Here's the drawing with two shaded views (mm, measured from the low corner). I have some questions. Coordinates: 2 decimals unless noted, no trailing zeros. Order: outer loops, then holes, each group sorted by start corner. A loop starts at its lowest first (then second) coordinate and runs counter-clockwise, first axis right, second up. Notation, with made-up numbers: (59, 65) -> (97, 65) arc R11 ccw to (97, 81) -> close; hole circle Ø4 at (13, 15). An arc over 180 degrees is marked (long way). Write item = value, one per line.
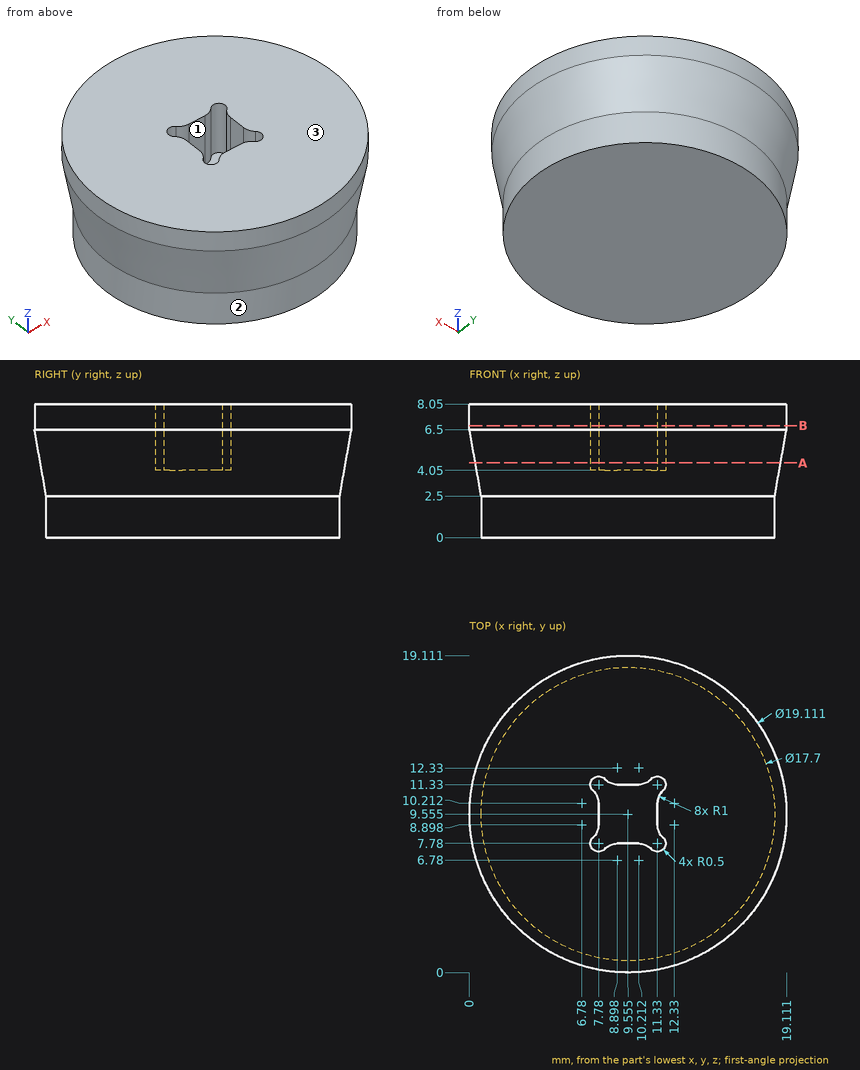
Item 1: I want a section at B-B, the plane z = 6.75. Please give me the cut outline in (x, y) (1 decimal).
A:
outline = circle Ø19.1 at (9.6, 9.6); hole (7.4, 8.2) arc R0.5 ccw (long way) to (8.2, 7.4) arc R1 cw to (8.9, 7.8) -> (10.2, 7.8) arc R1 cw to (11, 7.4) arc R0.5 ccw (long way) to (11.7, 8.2) arc R1 cw to (11.3, 8.9) -> (11.3, 10.2) arc R1 cw to (11.7, 11) arc R0.5 ccw (long way) to (11, 11.7) arc R1 cw to (10.2, 11.3) -> (8.9, 11.3) arc R1 cw to (8.2, 11.7) arc R0.5 ccw (long way) to (7.4, 11) arc R1 cw to (7.8, 10.2) -> (7.8, 8.9) arc R1 cw to start
Item 2: I'm going to push flat-ended pins straight in: P1, Ø3, axis at x = 17, z = 2.5, coming from the +Y side; P2, Ø1.1, axis at x = 9.5, z = 5, coming from the -Y side; P3, Ø1.5, axis at x = 4.5, z = 1, coming from the -Y side. Where does each tip first touch, or does it pass through?
A:
P1 = 16.16
P2 = 0.17
P3 = 1.82
Item 3: If I drill on probe 1 along X at (y, z) = (9.5, 4.75); probe 2 along X at (y, z) = (9.25, 4.5); probe 3 along Y at (x, z) = (11, 5) (1 decimal), over which ranges is the centre line in solid material (lowest first)?
A:
probe_1 = 0.31 to 7.78, 11.33 to 18.8
probe_2 = 0.36 to 7.78, 11.33 to 18.75
probe_3 = 0.4 to 7.4, 11.7 to 18.7
Item 4: I want a section at A-A, the plane z = 4.5. Please give me the cut outline in (x, y) (1 decimal).
A:
outline = circle Ø18.4 at (9.6, 9.6); hole (7.4, 8.2) arc R0.5 ccw (long way) to (8.2, 7.4) arc R1 cw to (8.9, 7.8) -> (10.2, 7.8) arc R1 cw to (11, 7.4) arc R0.5 ccw (long way) to (11.7, 8.2) arc R1 cw to (11.3, 8.9) -> (11.3, 10.2) arc R1 cw to (11.7, 11) arc R0.5 ccw (long way) to (11, 11.7) arc R1 cw to (10.2, 11.3) -> (8.9, 11.3) arc R1 cw to (8.2, 11.7) arc R0.5 ccw (long way) to (7.4, 11) arc R1 cw to (7.8, 10.2) -> (7.8, 8.9) arc R1 cw to start
Item 5: If we mould it in two halves opening along X, with no side actions, what happens to the marked faces 1, 2 and 3? For each: pulls with the +X half, pulls with the -X half, needs draft (parallel to the pull), parting line crosses it, or undercut.
A:
face_1 = undercut
face_2 = parting line crosses it
face_3 = needs draft
